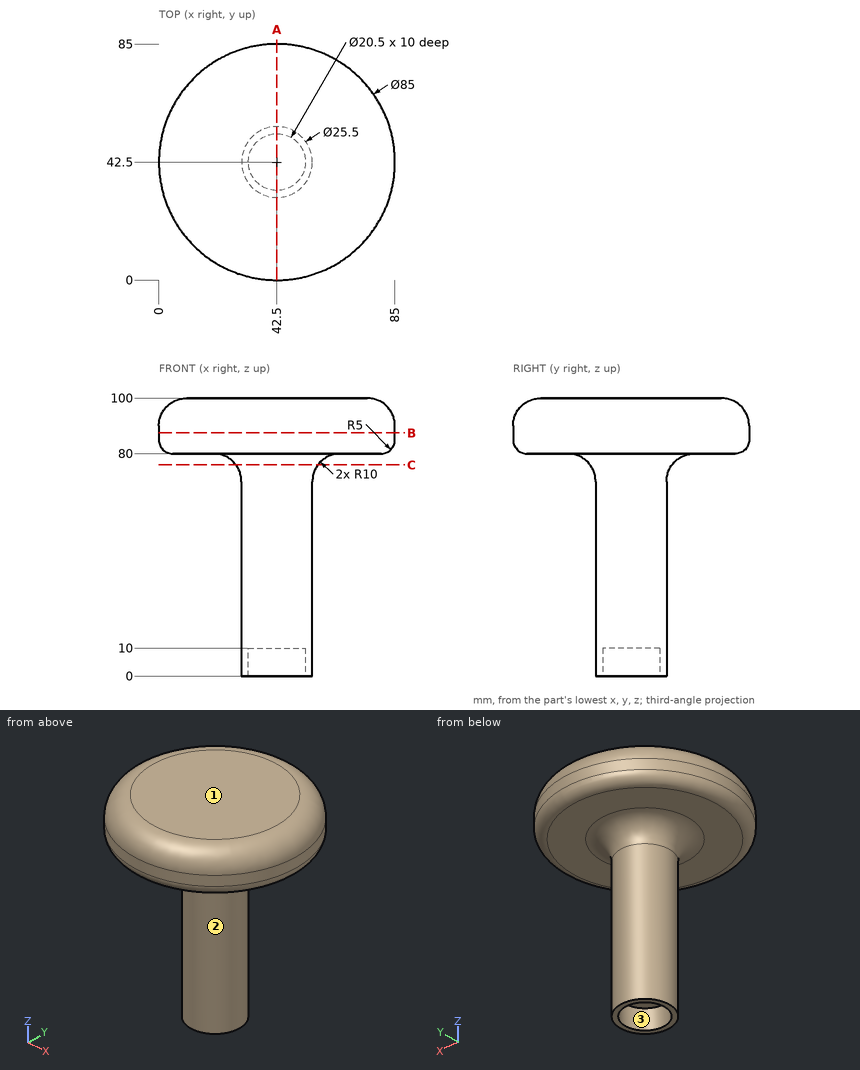
Source: three-view drawing plus pictorial views. Frame: mm from the lowest corner of the part. Round coordinates to 2 decimals unless told otherwise and drop trailing zeros. Loops run counter-clockwise (first coordinate to the right, second up) from the corner with the lowest first, then second, coordinate; pieces in that order, holes last. Notation, with made-up numbers: (-14, 61) - (-10, 61) arc R14 ccw to (-10, 83) - close; hole circle Ø9 at (38, 17). An arc over 180 degrees is marked (long way). Write item = value, one per line. Start each with the question number.
Item 1: Material intervals for line 1 (X direction, y = 42, z = 7); line 2 (Y direction, x = 42.5, z = 5.5); line 3 (Z direction, x = 13.5, y = 27), sorted ascending.
Item 2: Section query B-B on z = 87.5. Output: boundary loops of the cut face in (x, y).
Item 3: First-contact query: pin 1 Ø10 at (x, y) = (44, 39) entering from -Z; pin 2 Ø12 at (y, z) = (32, 10.5) entering from +X; pin 3 Ø4 at (x, z) = (45.5, 75) entering from +Y. Flat tips, straight axial feed; report the tip coordinate or a pass-through.
Item 4: Mould query, pull axis X, two halves, no side actions, for the marked faces 1, 2 and 3. Classes: released by +X, released by -X, zero draft, split by the parting line, or undercut.
Item 5: Section query A-A on x = 42.5. Output: boundary loops of the cut face in (y, z).
Item 6: Section query C-C on z = 76. Output: boundary loops of the cut face in (x, y), plus the area to 3 significant figures.
Results list:
q1.line_1 = 29.76 to 32.26, 52.74 to 55.24
q1.line_2 = 29.75 to 32.25, 52.75 to 55.25
q1.line_3 = 80 to 99.99
q2.outline = circle Ø85 at (42.5, 42.5)
q3.pin_1 = 10
q3.pin_2 = 54.43
q3.pin_3 = 57.85
q4.face_1 = zero draft
q4.face_2 = split by the parting line
q4.face_3 = undercut
q5.outline = (0, 85) arc R5 ccw to (5, 80) - (19.75, 80) arc R10 cw to (29.75, 70) - (29.75, 0) - (32.25, 0) - (32.25, 10) - (52.75, 10) - (52.75, 0) - (55.25, 0) - (55.25, 70) arc R10 cw to (65.25, 80) - (80, 80) arc R5 ccw to (85, 85) - (85, 90) arc R10 ccw to (75, 100) - (10, 100) arc R10 ccw to (0, 90) - close
q6.outline = circle Ø29.5 at (42.5, 42.5)
q6.area = 683 mm²
